Source: CAD feature listing. Evaluate the final solid. Frame: model axes, mm. Coordinates: 2 decimals unless noted, no trailing zeros. Write each loop counter-clockwise with the first axis right and the second up, starting at its lowest first coordinate (ties: lowest second). Pieces come first, ordered by that corner, then holes. Notation, with made-up numbers: (-12, -34) -> (41, -34) arc R30 ccw to (41, -3) -> close; hole circle Ø5 at (38.25, 7.25). An arc over 180 degrees is marked (long way). One line per item, written item: value. Start each with the question number.
1. Section query A-A, the plane y = 1.5. Output: boundary loops of the cut face in (x, z).
2. Line query: line 1 (Z direction, x = 1, y = 1.7); line 2 (Z direction, x = 15.3, y = 1.5); line 3 (X direction, y = 1.9, z = 42.5). Output: solid intervals per line, ascending.
3. Section query D-D, the plane z = 45. Output: boundary loops of the cut face in (x, y), and give its area (3 significant figures).
4. Section query C-C, the plane x = 0. Output: boundary loops of the cut face in (y, z).
5. Section query B-B, the plane z = -45. Output: boundary loops of the cut face in (x, y).
6. First-contact query: P1, Ø12, axis at x = 15.5, z = -34, coming from the +Y side; P2, Ø2, axis at y = 2.5, z = 36, coming from the +X side; P3, Ø1.2, axis at y = 2, z = 40, coming from the -X side; P4, Ø3, axis at y = 1.5, z = -45, coming from the -X side. Flat tips, straight axial feed; report the tip coordinate or a pass-through.
from build123d import *

# Parameters (mm, degrees)
BOSS_EXTRUDE1_DEPTH     = 3
BOSS_EXTRUDE2_START     = -10
SKETCH2_R               = 1.75
BOSS_EXTRUDE2_DEPTH     = 27.5
SKETCH3_W               = 8
SKETCH3_H               = 9
CUT_EXTRUDE1_DEPTH      = 24
SKETCH4_W               = 8
SKETCH4_H               = 9
CUT_EXTRUDE2_DEPTH      = 6.5
SKETCH5_W               = 7
SKETCH5_H               = 7
CUT_EXTRUDE3_DEPTH      = 14
CUT_EXTRUDE4_REACH      = 72.91
CUT_EXTRUDE4_END_RADIUS = 45.5
SKETCH6_W               = 11
SKETCH6_H               = 12


with BuildPart() as part:
    # Sketch1 → Boss-Extrude1 (new body)
    with BuildSketch(Plane(origin=(0, 0, 0), x_dir=(1, 0, 0), z_dir=(0, 1, 0))):
        with BuildLine():
            Line((-17.5, -42), (17.5, -42))
            ThreePointArc((17.5, -42), (45.5, 0), (17.5, 42))
            Line((17.5, 42), (-17.5, 42))
            ThreePointArc((-17.5, 42), (-45.5, 0), (-17.5, -42))
        make_face()
    extrude(amount=BOSS_EXTRUDE1_DEPTH)

    # Sketch2 → Boss-Extrude2 (add)
    with BuildSketch(Plane(origin=(0, 0, 0), x_dir=(0, 0, -1), z_dir=(1, 0, 0)).offset(BOSS_EXTRUDE2_START)):
        with BuildLine():
            Line((-42, 0), (-42.401923789, 0))
            ThreePointArc((-42.401923789, 0), (-48, 1.5), (-42.401923789, 3))
            Line((-42.401923789, 3), (-42, 3))
            Line((-42, 3), (-42, 1.5))
            Line((-42, 1.5), (-42, 0))
        make_face()
        with Locations((-45, 1.5)):
            Circle(SKETCH2_R, mode=Mode.SUBTRACT)
    boss_extrude2 = extrude(amount=BOSS_EXTRUDE2_DEPTH)

    # Mirror1: Boss-Extrude2 across plane
    add(boss_extrude2.mirror(Plane.XY))

    # Sketch3 → Cut-Extrude1 (cut)
    with BuildSketch(Plane.ZY.offset(10)):
        with Locations((46, 2)):
            Rectangle(SKETCH3_W, SKETCH3_H)
    extrude(amount=-CUT_EXTRUDE1_DEPTH, mode=Mode.SUBTRACT)

    # Sketch4 → Cut-Extrude2 (cut)
    with BuildSketch(Plane.ZY.offset(10)):
        with Locations((-46, 2)):
            Rectangle(SKETCH4_W, SKETCH4_H)
    extrude(amount=-CUT_EXTRUDE2_DEPTH, mode=Mode.SUBTRACT)

    # Sketch5 → Cut-Extrude3 (cut)
    with BuildSketch(Plane(origin=(17.5, 0, 0), x_dir=(0, 0, -1), z_dir=(1, 0, 0))):
        with Locations((45.5, 1.589580261)):
            Rectangle(SKETCH5_W, SKETCH5_H)
    extrude(amount=-CUT_EXTRUDE3_DEPTH, mode=Mode.SUBTRACT)

    # Cut-Extrude4: up to this cylinder (the profile starts inside it)
    cut_extrude4_end = Plane(origin=(0, 1.5, 0), z_dir=(0, -1, 0)) * Cylinder(CUT_EXTRUDE4_END_RADIUS, 237.82, mode=Mode.PRIVATE)
    # Sketch6 → Cut-Extrude4 (cut, up to the surface)
    with BuildSketch(Plane.ZY.offset(-6.5), mode=Mode.PRIVATE) as cut_extrude4_sk1:
        with Locations((45, 1.5)):
            Rectangle(SKETCH6_W, SKETCH6_H)
    cut_extrude4_tool1 = extrude(cut_extrude4_sk1.sketch, amount=CUT_EXTRUDE4_REACH, mode=Mode.PRIVATE) & cut_extrude4_end
    add(cut_extrude4_tool1.solids().sort_by_distance((6.5, 1.5, 45))[0], mode=Mode.SUBTRACT)


solid = part.part
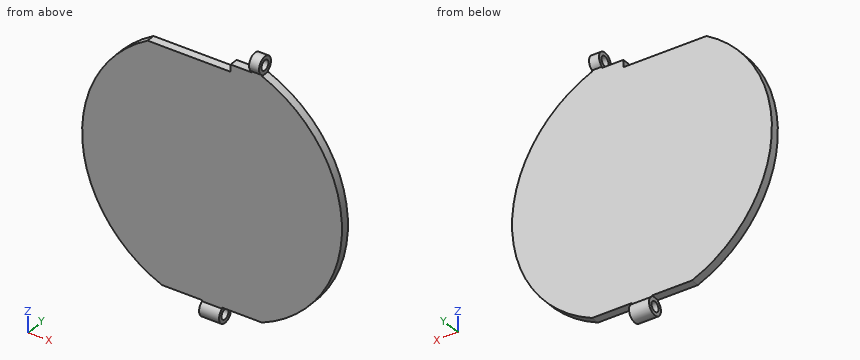
Computed values:
1. outline: (-22.58, 39.5) arc R45.5 ccw to (-17.5, -42) -> (-3.5, -42) -> (-3.5, -43.25) -> (3.5, -43.25) -> (3.5, -42) -> (17.5, -42) arc R45.5 ccw to (17.5, 42) -> (17.5, 43.25) -> (14, 43.25) -> (14, 42) -> (6.5, 42) -> (6.5, 39.5) -> close; (-3.5, -48) -> (3.5, -48) -> (3.5, -46.75) -> (-3.5, -46.75) -> close; (14, 46.75) -> (17.5, 46.75) -> (17.5, 48) -> (14, 48) -> close
2. line 1: z = -47.99 to -46.74, -43.26 to 39.5
2. line 2: z = -42 to 43.25, 46.75 to 48
2. line 3: x = 14 to 17.5
3. outline: (14, -1.5) -> (17.5, -1.5) -> (17.5, -0.25) -> (14, -0.25) -> close; (14, 3.25) -> (17.5, 3.25) -> (17.5, 4.5) -> (14, 4.5) -> close
3. area: 8.75 mm²
4. outline: (0, -42.4) arc R3 ccw (long way) to (3, -42.4) -> (3, 39.5) -> (0, 39.5) -> close; hole circle Ø3.5 at (1.5, -45)
5. outline: (-3.5, -1.5) -> (3.5, -1.5) -> (3.5, -0.25) -> (-3.5, -0.25) -> close; (-3.5, 3.25) -> (3.5, 3.25) -> (3.5, 4.5) -> (-3.5, 4.5) -> close
6. P1: stops at y = 3
6. P2: stops at x = 29.07
6. P3: stops at x = -22.76
6. P4: passes through
